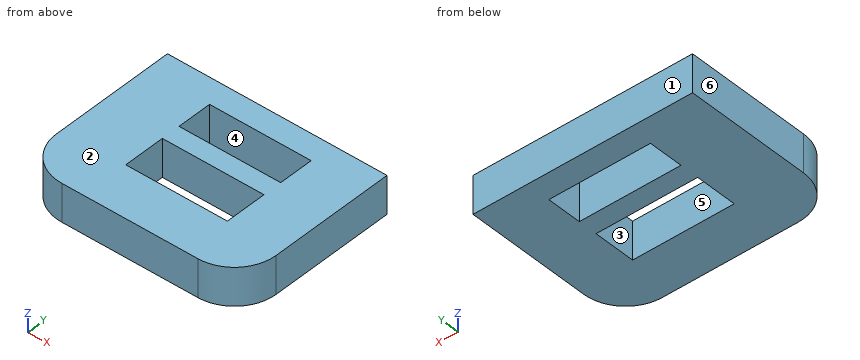
from build123d import *

# Parameters (mm, degrees)
SKETCH1_W           = 7.305190172
SKETCH1_H           = 3
SKETCH1_H_2         = 2.5
BOSS_EXTRUDE1_DEPTH = 2.719448


with BuildPart() as part:
    # Sketch1 → Boss-Extrude1 (new body)
    with BuildSketch(Plane.XY):
        with BuildLine():
            Line((-25.252187622, -417.522040931), (-35.0337538, -417.522040931))
            ThreePointArc((-35.0337538, -417.522040931), (-37.155074144, -416.643361274), (-38.0337538, -414.522040931))
            Line((-38.0337538, -414.522040931), (-38.0337538, -405.428571358))
            Line((-38.0337538, -405.428571358), (-22.252187622, -405.428571358))
            Line((-22.252187622, -405.428571358), (-22.252187622, -414.522040931))
            ThreePointArc((-22.252187622, -414.522040931), (-23.130867278, -416.643361274), (-25.252187622, -417.522040931))
        make_face()
        with Locations((-29.82012001, -412.555740742)):
            Rectangle(SKETCH1_W, SKETCH1_H, mode=Mode.SUBTRACT)
        with Locations((-29.82012001, -408.432910126)):
            Rectangle(SKETCH1_W, SKETCH1_H_2, mode=Mode.SUBTRACT)
    extrude(amount=BOSS_EXTRUDE1_DEPTH)


solid = part.part
Can you work these out from the model? Positions are in its coordinate system, mm. Face numbers are marked on the shaded views. A direction names the side the tool comes from. Coordinates: 2 decimals unless noted, no trailing zeros. Order: outer loops, then holes, each group sorted by start corner. A loop starts at its lowest first (then second) coordinate and runs counter-clockwise, first axis right, second up. Notation, with made-up numbers: (-20, 2) - (32, 2) arc R13 cw to (32, 17) - close; hole circle Ø8 at (78.5, -37). An arc over 180 degrees is marked (long way). Answer as a JSON object with one key per item and string values. Group by question number.
Q1. Imagine slicing it at B-B (y = -409.5). Please give me the cut outline in (x, z), and give its area (3 significant figures).
Q2. On a 3-axis mill with a long thin cutter (end or side, diameter ignored), from which of +Z, -Z, +X, -X, +Y, -Y can I reach the whole of each face in a straight line? I mean the marked faces 5 and 6. Say none if no direction works.
Q3. Will this pin go through, and if not, where does the flat tip stop? P1, Ø1, axis at x = -32, y = -407.5, coming from the -Z side.
Q4. Imagine slicing it at A-A (x = -29.25). Please give me the cut outline in (y, z), and give its area (3 significant figures).
Q5. We'd pull the mould along Y, two halves only. Please class the marked faces 1, 2, 3 and 4: +Y half, -Y half, draft (parallel to the pull), parting line (faces both ways), or undercut.
Q6. Imagine slicing it at C-C (z = 0.85). Please give me the cut outline in (x, y).
Q7. I need wall thicknesses on line 1 (Y direction, x = -28.5, z = 1.5); line 2 (X direction, y = -411.75, z = 1.85); line 3 (X direction, y = -416, z = 0.1). Which ranges of each line are inside material? Lowest first, please. Write a range as from..to.
Determined:
{
 "1": {"outline": "(-38.03, 0) - (-33.47, 0) - (-33.47, 2.72) - (-38.03, 2.72) - close; (-26.17, 0) - (-22.25, 0) - (-22.25, 2.72) - (-26.17, 2.72) - close", "area": "23.1 mm2"},
 "2": {"face 5": "+Z, -Z", "face 6": "+Z, -Z, -X, +Y, -Y"},
 "3": {"P1": "stops at z = 0"},
 "4": {"outline": "(-417.52, 0) - (-414.06, 0) - (-414.06, 2.72) - (-417.52, 2.72) - close; (-411.06, 0) - (-409.68, 0) - (-409.68, 2.72) - (-411.06, 2.72) - close; (-407.18, 0) - (-405.43, 0) - (-405.43, 2.72) - (-407.18, 2.72) - close", "area": "17.9 mm2"},
 "5": {"face 1": "+Y half", "face 2": "draft", "face 3": "undercut", "face 4": "undercut"},
 "6": {"outline": "(-38.03, -414.52) arc R3 ccw to (-35.03, -417.52) - (-25.25, -417.52) arc R3 ccw to (-22.25, -414.52) - (-22.25, -405.43) - (-38.03, -405.43) - close; hole (-33.47, -414.06) - (-26.17, -414.06) - (-26.17, -411.06) - (-33.47, -411.06) - close; hole (-33.47, -409.68) - (-26.17, -409.68) - (-26.17, -407.18) - (-33.47, -407.18) - close"},
 "7": {"line 1": "y = -417.52..-414.06, -411.06..-409.68, -407.18..-405.43", "line 2": "x = -38.03..-33.47, -26.17..-22.25", "line 3": "x = -37.64..-22.64"}
}
